```python
from build123d import *

# Parameters (mm, degrees)
BOSS_EXTRUDE2_DEPTH = 0.1778


with BuildPart() as part:
    # Sketch1 → Boss-Extrude2 (new body)
    with BuildSketch(Plane.XY):
        with BuildLine():
            Line((28.466511978, 5.161354222), (28.466511978, 15.161354222))
            ThreePointArc((28.466511978, 15.161354222), (28.344498508, 16.400177767), (27.983147009, 17.591394018))
            Line((27.983147009, 17.591394018), (22.910261978, 29.838421861))
            Line((22.910261978, 29.838421861), (21.322761978, 29.838421861))
            Line((21.322761978, 29.838421861), (16.249876946, 17.591394018))
            ThreePointArc((16.249876946, 17.591394018), (15.888525447, 16.400177767), (15.766511978, 15.161354222))
            Line((15.766511978, 15.161354222), (15.766511978, 5.161354222))
            ThreePointArc((15.766511978, 5.161354222), (22.116511978, -1.188645778), (28.466511978, 5.161354222))
        make_face()
    extrude(amount=-BOSS_EXTRUDE2_DEPTH)


solid = part.part
```
Can you work these out from the model? Positions are in its coordinate system, mm. Coordinates: 2 decimals unless noted, no trailing zeros. Loops run counter-clockwise (first coordinate to the right, second up) from the corner with the lowest first, then second, coordinate; pieces in that order, holes last. Notation, with made-up numbers: M 86,-29 L 139,-29 A13 cw 139,-4 Z; hole C 43,0 d1. An arc over 180 degrees is marked long. Put each result on its own line as item: value. Start each with the question number.
(1) Imagine slicing it at C-C on y = 21. List the corners of the cut face in (x, z) for me.
(2) Will this pin go through, and if not, where does the flat tip stop? pin 1 Ø1 at (x, y) = (17.5, 11) entering from +Z.
(3) I need wall thicknesses on probe 1 along X at (y, z) = (27, -0.1); probe 2 along Y at (x, z) = (25.5, -0.05); probe 3 along X at (y, z) = (24, -0.1). Which ranges of each line are inside material? Lowest first, please.
(4) Imagine slicing it at B-B on x = 19.5. List the corners of the cut face in (y, z) for me, and give its area (3 significant figures).
(5) Imagine slicing it at A-A on z = -0.1. List the corners of the cut face in (x, y) for me.
Worked answers:
1. outline: M 17.66,-0.18 L 26.57,-0.18 L 26.57,0 L 17.66,0 Z
2. pin 1: stops at z = 0
3. probe 1: x = 20.15 to 24.09
3. probe 2: y = -0.21 to 23.59
3. probe 3: x = 18.9 to 25.33
4. outline: M -0.62,-0.18 L 25.44,-0.18 L 25.44,0 L -0.62,0 Z
4. area: 4.63 mm2
5. outline: M 15.77,5.16 A6.35 ccw 28.47,5.16 L 28.47,15.16 A6.35 ccw 27.98,17.59 L 22.91,29.84 L 21.32,29.84 L 16.25,17.59 A6.35 ccw 15.77,15.16 Z
